from build123d import *

# Parameters (mm, degrees)
F1_DEPTH  = 50.8
F2_W      = 12.7
F2_H      = 25.4
F3_DEPTH  = 69.85
F5_DEPTH  = 12.7
F6_DEPTH  = 25.4
F7_R      = 6.35
F8_DEPTH  = 25.4
F9_W      = 12.7
F9_H      = 12.7
F10_DEPTH = 12.7
F11_W     = 12.7
F11_H     = 12.7
F12_DEPTH = 12.7
F14_DEPTH = 25.4
F15_R     = 3.175
F16_DEPTH = 25.4
F18_DEPTH = 25.4


with BuildPart() as f1:
    # F0 (on Right) → F1 (new body)
    with BuildSketch(Plane.YZ):
        Polygon((-31.75, 0), (0, 0), (0, 76.2), (-25.4, 76.2), (-25.4, 50.8), (-12.7, 50.8), (-12.7, 6.35), (-31.75, 6.35), align=None)
    extrude(amount=F1_DEPTH)

    # F2 (on face) → F3 (cut)
    with BuildSketch(Plane.XY.offset(76.2)):
        with Locations((6.35, -12.7)):
            Rectangle(F2_W, F2_H)
        with Locations((44.45, -12.7)):
            Rectangle(F2_W, F2_H)
    extrude(amount=-F3_DEPTH, mode=Mode.SUBTRACT)

    # F4 (on face) → F5 (cut)
    with BuildSketch(Plane.XZ.offset(25.4)):
        with BuildLine():
            ThreePointArc((12.7, 63.5), (16.4197438789, 72.4802561211), (25.4, 76.2))
            Line((25.4, 76.2), (12.7, 76.2))
            Line((12.7, 76.2), (12.7, 63.5))
        make_face()
        with BuildLine():
            ThreePointArc((25.4, 76.2), (34.3802561211, 72.4802561211), (38.1, 63.5))
            Line((38.1, 63.5), (38.1, 76.2))
            Line((38.1, 76.2), (25.4, 76.2))
        make_face()
        with BuildLine():
            Line((12.7, 50.8), (25.4, 50.8))
            ThreePointArc((25.4, 50.8), (16.4197438789, 54.5197438789), (12.7, 63.5))
            Line((12.7, 63.5), (12.7, 50.8))
        make_face()
        with BuildLine():
            Line((38.1, 50.8), (38.1, 63.5))
            ThreePointArc((38.1, 63.5), (34.3802561211, 54.5197438789), (25.4, 50.8))
            Line((25.4, 50.8), (38.1, 50.8))
        make_face()
    extrude(amount=-F5_DEPTH, mode=Mode.SUBTRACT)

    # F6 (cut): faces of the model
    f6_faces = [f1.faces().sort_by_distance(p)[0] for p in [
        (15.5367728246, -12.7, 73.3632271754),
        (35.2632271754, -12.7, 73.3632271754),
    ]]
    extrude(f6_faces, amount=-F6_DEPTH, mode=Mode.SUBTRACT)

    # F7 (on face) → F8 (cut)
    with BuildSketch(Plane.XZ.offset(25.4)):
        with Locations((25.4, 63.5)):
            Circle(F7_R)
    extrude(amount=-F8_DEPTH, mode=Mode.SUBTRACT)

    # F9 (on face) → F10 (join)
    with BuildSketch(Plane(origin=(12.7, 0, 0), x_dir=(0, -1, 0), z_dir=(-1, 0, 0))):
        with Locations((6.35, 12.7)):
            Rectangle(F9_W, F9_H)
    extrude(amount=F10_DEPTH)

    # F11 (on face) → F12 (join)
    with BuildSketch(Plane.YZ.offset(38.1)):
        with Locations((-6.35, 12.7)):
            Rectangle(F11_W, F11_H)
    extrude(amount=F12_DEPTH)

    # F13 (on face) → F14 (cut)
    with BuildSketch(Plane.XZ.offset(12.7)):
        with BuildLine():
            ThreePointArc((0, 6.35), (8.9802561211, 10.0697438789), (12.7, 19.05))
            Line((12.7, 19.05), (0, 19.05))
            Line((0, 19.05), (0, 6.35))
        make_face()
        with BuildLine():
            ThreePointArc((38.1, 19.05), (41.8197438789, 10.0697438789), (50.8, 6.35))
            Line((50.8, 6.35), (50.8, 19.05))
            Line((50.8, 19.05), (38.1, 19.05))
        make_face()
    extrude(amount=-F14_DEPTH, mode=Mode.SUBTRACT)

    # F15 (on face) → F16 (cut)
    with BuildSketch(Plane.XY.offset(6.35)):
        with Locations((9.525, -22.225)):
            Circle(F15_R)
        with Locations((41.275, -22.225)):
            Circle(F15_R)
    extrude(amount=-F16_DEPTH, mode=Mode.SUBTRACT)

    # F17 (on face) → F18 (cut)
    with BuildSketch(Plane.XY.offset(6.35)):
        with BuildLine():
            Line((0, -31.75), (6.35, -31.75))
            ThreePointArc((6.35, -31.75), (1.8598719395, -29.8901280605), (0, -25.4))
            Line((0, -25.4), (0, -31.75))
        make_face()
        with BuildLine():
            ThreePointArc((50.8, -25.4), (48.9401280605, -29.8901280605), (44.45, -31.75))
            Line((44.45, -31.75), (50.8, -31.75))
            Line((50.8, -31.75), (50.8, -25.4))
        make_face()
    extrude(amount=-F18_DEPTH, mode=Mode.SUBTRACT)


solid = f1.part
Design review of the part built by this model. Coordinates are the model's own, in mm. A direction names the side the tool comes from. Coordinates: 2 decimals unless noted, no trailing zeros. Order: outer loops, then holes, each group sorted by start corner. A loop starts at its lowest first (then second) coordinate and runs counter-clockwise, first axis right, second up. Notation, with made-up numbers: (50, -33.5) -> (75, -33.5) arc R25 cw to (75, 4.5) -> close; hole circle Ø7 at (64, 41). An arc over 180 degrees is marked (long way). One line per item, written item: value.
1) We need section D-D, the plane z = 27. Give the boundary of the cut face in (x, y).
Output values:
outline: (12.7, -12.7) -> (38.1, -12.7) -> (38.1, 0) -> (12.7, 0) -> close
2) Draft analysis for pull direction Z (two halves, no side actions). For faces 5 (the face through (8.88, -6.44, 9.97)), 6 (the face through (31.26, -15.7, 74.767)), 7 (the face through (25, -16, 0)), state which applies: +Z half, -Z half, draft (parallel to the pull), parting line (faces both ways), or undercut.
Output values:
face 5: +Z half
face 6: undercut
face 7: -Z half
3) Clearance check with flat-ended pins moving along their axes: P1, Ø2, axis at y = -10, z = 57, coming from the +X side; P2, Ø7.5, axis at x = 23.5, z = 69, coming from the -Y side; P3, Ø6, axis at y = -21, z = 65, coming from the -X side; P4, Ø10, axis at x = 25.4, z = 63.5, coming from the -Y side. State where each tip first meets the part, or that it passes through.
Output values:
P1: stops at x = 38.1
P2: stops at y = -25.4
P3: stops at x = 12.7
P4: passes through
4) To check wall thickness, follow probe 1 along X at (y, z) = (-11, 63); probe 2 along Z at (x, y) = (25.4, -14); probe 3 along Z at (x, y) = (27, -18.5). State the ranges of each line that lie inside material, in increasing order. Write a range as [from, to].
Output values:
probe 1: x = [12.7, 19.07], [31.73, 38.1]
probe 2: z = [0, 6.35], [50.8, 57.15], [69.85, 76.2]
probe 3: z = [0, 6.35], [50.9, 57.35], [69.65, 76.1]
5) We need section B-B, the plane x = 25.4. Give the boundary of the cut face in (y, z).
Output values:
outline: (-31.75, 0) -> (0, 0) -> (0, 57.15) -> (-25.4, 57.15) -> (-25.4, 50.8) -> (-12.7, 50.8) -> (-12.7, 6.35) -> (-31.75, 6.35) -> close; (-25.4, 69.85) -> (0, 69.85) -> (0, 76.2) -> (-25.4, 76.2) -> close
6) We need section C-C, the plane y = -8. Give the boundary of the cut face in (x, z).
Output values:
outline: (0, 0) -> (50.8, 0) -> (50.8, 6.35) arc R12.7 cw to (38.1, 19.05) -> (38.1, 63.5) arc R12.7 ccw to (12.7, 63.5) -> (12.7, 19.05) arc R12.7 cw to (0, 6.35) -> close; hole circle Ø12.7 at (25.4, 63.5)
7) We need section A-A, the plane y = -18. Give the boundary of the cut face in (x, z), then the cut area to 3 significant figures.
Output values:
outline: (0, 0) -> (50.8, 0) -> (50.8, 6.35) -> (0, 6.35) -> close; circle Ø25.4 at (25.4, 63.5); hole circle Ø12.7 at (25.4, 63.5)
area: 703 mm2
8) Machinability: for faces 1 (the face through (38.1, -6, 42)), 2 (the face through (25, -22, 6.35)), 3 (the face through (22.4, -25.4, 69.3)), 4 (the face through (12.7, -6, 42)), which of the approach directions +Z, -Z, +X, -X, +Y, -Y give a long, thin tool a straight path to every point of the face, cutting with its end or side? Answer none if there is none.
Output values:
face 1: +Z, +X, +Y, -Y
face 2: +X, -X, -Y
face 3: +Z, +X, -X, -Y
face 4: +Z, -X, +Y, -Y
